```python
from build123d import *

# Parameters (mm, degrees)
SKETCH2_R          = 4
CUT_EXTRUDE1_DEPTH = 39.594040991
SKETCH3_R          = 1.5
CUT_EXTRUDE2_DEPTH = 39.594040991
CIRPATTERN1_COUNT  = 2
CIRPATTERN1_ANGLE  = 90
CUT_EXTRUDE3_DEPTH = 26
FILLET2_R          = 1
CIRPATTERN2_START  = 1.5
CIRPATTERN2_DEPTH  = 26


# Read off the part's stored shape, not the designer's step: CirPattern2
with BuildPart() as part:
    # Sketch1 → Revolve1 (revolve)
    with BuildSketch(Plane.XY, mode=Mode.PRIVATE) as revolve1_sk:
        Polygon((0, 0), (0, 11.5), (1.5, 11.5), (1.5, 9.5), (27.5, 9.5), (27.5, 11.5), (29, 11.5), (29, 6.5), (35, 6.5), (35, 0), align=None)
    revolve(revolve1_sk.sketch.rotate(Axis((-4.735156117, 0, 0), (1, 0, 0)), 90), axis=Axis((-4.735156117, 0, 0), (1, 0, 0)))

    # Sketch2 → Cut-Extrude1 (cut, through all)
    with BuildSketch(Plane.ZY):
        Circle(SKETCH2_R)
    extrude(amount=-CUT_EXTRUDE1_DEPTH, mode=Mode.SUBTRACT)

    # Sketch3 → Cut-Extrude2 (cut, through all)
    with BuildSketch(Plane(origin=(0, 0, 0), x_dir=(1, 0, 0), z_dir=(0, 1, 0))):
        with Locations(Location((32, 0, 0), (0, 0, 90))):
            Circle(SKETCH3_R)
    cut_extrude2 = extrude(amount=CUT_EXTRUDE2_DEPTH, mode=Mode.SUBTRACT)

    # CirPattern1: Cut-Extrude2 ×2 about axis
    cirpattern1_axis = Axis((-4.735156117, 0, 0), (-1, 0, 0))
    for i in range(1, CIRPATTERN1_COUNT):
        add(cut_extrude2.rotate(cirpattern1_axis, i * CIRPATTERN1_ANGLE / (CIRPATTERN1_COUNT - 1)), mode=Mode.SUBTRACT)

    # Sketch4 → Cut-Extrude3 (cut)
    with BuildSketch(Plane(origin=(1.5, 0, 0), x_dir=(0, 0, -1), z_dir=(1, 0, 0))):
        Polygon((2, 11.5), (-2, 11.5), (-1, 7.5), (1, 7.5), align=None)
    extrude(amount=CUT_EXTRUDE3_DEPTH, mode=Mode.SUBTRACT)

    # Fillet2
    fillet2_edges = [part.edges().sort_by_distance(p)[0] for p in [
        (14.5, 7.5, -1),
        (14.5, 9.385369037, -1.471342259),
        (14.5, 9.385369037, 1.471342259),
        (14.5, 7.5, 1),
    ]]
    fillet(fillet2_edges, radius=FILLET2_R)

    # CirPattern2 outline → CirPattern2 (cut)
    with BuildSketch(Plane.YZ.offset(CIRPATTERN2_START)):
        with BuildLine():
            ThreePointArc((9.173931529, 2.467585925), (8.227241336, 4.75), (6.723957861, 6.711064794))
            ThreePointArc((6.723957861, 6.711064794), (7.00459855, 5.999230542), (6.6998571, 5.297375964))
            Line((6.6998571, 5.297375964), (6.556490873, 5.158753439))
            ThreePointArc((6.556490873, 5.158753439), (6.261292098, 4.578713089), (6.385578732, 3.939853201))
            Line((6.385578732, 3.939853201), (6.604802325, 3.560146799))
            ThreePointArc((6.604802325, 3.560146799), (7.095927901, 3.133081473), (7.745856966, 3.098710936))
            Line((7.745856966, 3.098710936), (7.937590709, 3.153558469))
            ThreePointArc((7.937590709, 3.153558469), (8.697785327, 3.066545017), (9.173931529, 2.467585925))
        make_face()
        with BuildLine():
            ThreePointArc((6.723957861, 6.711064794), (4.757893172, 8.22267916), (2.467585925, 9.173931529))
            ThreePointArc((2.467585925, 9.173931529), (3.066545017, 8.697785327), (3.153558469, 7.937590709))
            Line((3.153558469, 7.937590709), (3.098710936, 7.745856966))
            ThreePointArc((3.098710936, 7.745856966), (3.133081473, 7.095927901), (3.560146799, 6.604802325))
            Line((3.560146799, 6.604802325), (3.939853201, 6.385578732))
            ThreePointArc((3.939853201, 6.385578732), (4.578713089, 6.261292098), (5.158753439, 6.556490873))
            Line((5.158753439, 6.556490873), (5.297272586, 6.699750184))
            ThreePointArc((5.297272586, 6.699750184), (6.008242375, 7.004605475), (6.723957861, 6.711064794))
        make_face()
        with BuildLine():
            ThreePointArc((2.467585925, 9.173931529), (0.009116775, 9.499995625), (-2.449973668, 9.178650719))
            ThreePointArc((-2.449973668, 9.178650719), (-1.693186777, 9.065775559), (-1.237733608, 8.450934433))
            Line((-1.237733608, 8.450934433), (-1.189366094, 8.257464375))
            ThreePointArc((-1.189366094, 8.257464375), (-0.834635803, 7.711794562), (-0.219223594, 7.5))
            Line((-0.219223594, 7.5), (0.219223594, 7.5))
            ThreePointArc((0.219223594, 7.5), (0.834635803, 7.711794562), (1.189366094, 8.257464375))
            Line((1.189366094, 8.257464375), (1.237697538, 8.450790151))
            ThreePointArc((1.237697538, 8.450790151), (1.700987791, 9.070287472), (2.467585925, 9.173931529))
        make_face()
        with BuildLine():
            ThreePointArc((-2.449973668, 9.178650719), (-4.742102454, 8.231795935), (-6.711064795, 6.723957862))
            ThreePointArc((-6.711064795, 6.723957862), (-5.999230542, 7.00459855), (-5.297375964, 6.6998571))
            Line((-5.297375964, 6.6998571), (-5.158753439, 6.556490873))
            ThreePointArc((-5.158753439, 6.556490873), (-4.578713089, 6.261292098), (-3.939853201, 6.385578732))
            Line((-3.939853201, 6.385578732), (-3.560146799, 6.604802325))
            ThreePointArc((-3.560146799, 6.604802325), (-3.133081473, 7.095927901), (-3.098710936, 7.745856966))
            Line((-3.098710936, 7.745856966), (-3.153517566, 7.937447722))
            ThreePointArc((-3.153517566, 7.937447722), (-3.062045097, 8.705593266), (-2.449973668, 9.178650719))
        make_face()
        with BuildLine():
            ThreePointArc((-6.711064795, 6.723957862), (-8.22267916, 4.757893172), (-9.173931529, 2.467585925))
            ThreePointArc((-9.173931529, 2.467585925), (-8.697785327, 3.066545017), (-7.937590709, 3.153558469))
            Line((-7.937590709, 3.153558469), (-7.745856966, 3.098710936))
            ThreePointArc((-7.745856966, 3.098710936), (-7.095927901, 3.133081473), (-6.604802325, 3.560146799))
            Line((-6.604802325, 3.560146799), (-6.385578732, 3.939853201))
            ThreePointArc((-6.385578732, 3.939853201), (-6.261292098, 4.578713089), (-6.556490873, 5.158753439))
            Line((-6.556490873, 5.158753439), (-6.699750184, 5.297272586))
            ThreePointArc((-6.699750184, 5.297272586), (-7.004605475, 6.008242375), (-6.711064795, 6.723957862))
        make_face()
        with BuildLine():
            ThreePointArc((-9.173931529, 2.467585925), (-9.499995625, 0.009116775), (-9.178650719, -2.449973668))
            ThreePointArc((-9.178650719, -2.449973668), (-9.065775559, -1.693186777), (-8.450934433, -1.237733608))
            Line((-8.450934433, -1.237733608), (-8.257464375, -1.189366094))
            ThreePointArc((-8.257464375, -1.189366094), (-7.711794562, -0.834635803), (-7.5, -0.219223594))
            Line((-7.5, -0.219223594), (-7.5, 0.219223594))
            ThreePointArc((-7.5, 0.219223594), (-7.711794562, 0.834635803), (-8.257464375, 1.189366094))
            Line((-8.257464375, 1.189366094), (-8.450790151, 1.237697538))
            ThreePointArc((-8.450790151, 1.237697538), (-9.070287472, 1.700987791), (-9.173931529, 2.467585925))
        make_face()
        with BuildLine():
            ThreePointArc((-9.178650719, -2.449973668), (-8.231795935, -4.742102454), (-6.723957862, -6.711064795))
            ThreePointArc((-6.723957862, -6.711064795), (-7.00459855, -5.999230542), (-6.6998571, -5.297375964))
            Line((-6.6998571, -5.297375964), (-6.556490873, -5.158753439))
            ThreePointArc((-6.556490873, -5.158753439), (-6.261292098, -4.578713089), (-6.385578732, -3.939853201))
            Line((-6.385578732, -3.939853201), (-6.604802325, -3.560146799))
            ThreePointArc((-6.604802325, -3.560146799), (-7.095927901, -3.133081473), (-7.745856966, -3.098710936))
            Line((-7.745856966, -3.098710936), (-7.937447722, -3.153517566))
            ThreePointArc((-7.937447722, -3.153517566), (-8.705593266, -3.062045097), (-9.178650719, -2.449973668))
        make_face()
        with BuildLine():
            ThreePointArc((-6.723957862, -6.711064795), (-4.757893172, -8.22267916), (-2.467585925, -9.173931529))
            ThreePointArc((-2.467585925, -9.173931529), (-3.066545017, -8.697785327), (-3.153558469, -7.937590709))
            Line((-3.153558469, -7.937590709), (-3.098710936, -7.745856966))
            ThreePointArc((-3.098710936, -7.745856966), (-3.133081473, -7.095927901), (-3.560146799, -6.604802325))
            Line((-3.560146799, -6.604802325), (-3.939853201, -6.385578732))
            ThreePointArc((-3.939853201, -6.385578732), (-4.578713089, -6.261292098), (-5.158753439, -6.556490873))
            Line((-5.158753439, -6.556490873), (-5.297272586, -6.699750184))
            ThreePointArc((-5.297272586, -6.699750184), (-6.008242375, -7.004605475), (-6.723957862, -6.711064795))
        make_face()
        with BuildLine():
            ThreePointArc((-2.467585925, -9.173931529), (-0.009116775, -9.499995625), (2.449973668, -9.178650719))
            ThreePointArc((2.449973668, -9.178650719), (1.693186777, -9.065775559), (1.237733608, -8.450934433))
            Line((1.237733608, -8.450934433), (1.189366094, -8.257464375))
            ThreePointArc((1.189366094, -8.257464375), (0.834635803, -7.711794562), (0.219223594, -7.5))
            Line((0.219223594, -7.5), (-0.219223594, -7.5))
            ThreePointArc((-0.219223594, -7.5), (-0.834635803, -7.711794562), (-1.189366094, -8.257464375))
            Line((-1.189366094, -8.257464375), (-1.237697538, -8.450790151))
            ThreePointArc((-1.237697538, -8.450790151), (-1.700987791, -9.070287472), (-2.467585925, -9.173931529))
        make_face()
        with BuildLine():
            ThreePointArc((2.449973668, -9.178650719), (4.742102454, -8.231795935), (6.711064794, -6.723957861))
            ThreePointArc((6.711064794, -6.723957861), (5.999230542, -7.00459855), (5.297375964, -6.6998571))
            Line((5.297375964, -6.6998571), (5.158753439, -6.556490873))
            ThreePointArc((5.158753439, -6.556490873), (4.578713089, -6.261292098), (3.939853201, -6.385578732))
            Line((3.939853201, -6.385578732), (3.560146799, -6.604802325))
            ThreePointArc((3.560146799, -6.604802325), (3.133081473, -7.095927901), (3.098710936, -7.745856966))
            Line((3.098710936, -7.745856966), (3.153517566, -7.937447722))
            ThreePointArc((3.153517566, -7.937447722), (3.062045097, -8.705593266), (2.449973668, -9.178650719))
        make_face()
        with BuildLine():
            Line((6.556490873, -5.158753439), (6.699750184, -5.297272586))
            ThreePointArc((6.699750184, -5.297272586), (7.004605475, -6.008242375), (6.711064795, -6.723957862))
            ThreePointArc((6.711064795, -6.723957862), (8.22267916, -4.757893172), (9.173931529, -2.467585925))
            ThreePointArc((9.173931529, -2.467585925), (8.697785327, -3.066545017), (7.937590709, -3.153558469))
            Line((7.937590709, -3.153558469), (7.745856966, -3.098710936))
            ThreePointArc((7.745856966, -3.098710936), (7.095927901, -3.133081473), (6.604802325, -3.560146799))
            Line((6.604802325, -3.560146799), (6.385578732, -3.939853201))
            ThreePointArc((6.385578732, -3.939853201), (6.261292098, -4.578713089), (6.556490873, -5.158753439))
        make_face()
    extrude(amount=CIRPATTERN2_DEPTH, mode=Mode.SUBTRACT)


solid = part.part
```
Part model, mm, in its own coordinate system. A direction names the side the tool comes from. Round coordinates to 2 decimals unless told otherwise and drop trailing zeros. Loops run counter-clockwise (first coordinate to the right, second up) from the corner with the lowest first, then second, coordinate; pieces in that order, holes last. Notation, with made-up numbers: (-22.5, -13.75) -> (-18.5, -13.75) arc R23 ccw to (-18.5, 10.25) -> close; hole circle Ø6 at (-27, 28.25). An arc over 180 degrees is marked (long way). Use one line per item in the form item = value. Start each with the question number.
Item 1: Band-saw the part on C-C (z = 4.5). List the corners of the cut face in (x, y), plus the area to 3 significant figures.
Item 2: Band-saw the part on A-A (y = 10.25). List the corners of the cut face in (x, z).
Item 3: Band-saw the part on B-B (x = 32). List the corners of the cut face in (y, z), plus the area to 3 significant figures.
Item 4: Tool access for faces 4 (the cylindrical face through (14.318, 7.087, 3.137)), 5 (the cylindrical face through (14.318, -8.696, -3.067)), 6 (the cylindrical face through (14.32, -7.71, 0.83)): list every direction of +Z, -Z, +X, -X, +Y, -Y with a clear straight run to the whole face (end or side of a thin tool).
Item 5: Drop flat-ended pins along their axis: pin 1 Ø5 at (x, y) = (32, 0) entering from -Z; pin 2 Ø1.5 at (x, y) = (22.5, 6.5) entering from +Z; pin 3 Ø1.5 at (x, y) = (29.5, 1.5) entering from +Z; pin 4 Ø11.5 at (y, z) = (-2, 2) entering from -X. Give the stop position or say it passes through.
Item 6: Drill centre lines: line 1 along Z through (x, y) = (21.5, 0); line 2 along X through (y, z) = (4.4, 0); line 3 along X through (y, z) = (8.5, -6). Where is each one in solid material? Low to high.
Item 7: Two-plate mould, pull along X, no slides. Class faces 1 (the flat face through (0, 0, -5)), 2 (the cylindrical face through (14.318, -6.01, 7.005)), 3 (the cylindrical face through (0.8, -11.4, -1.5)): released by +X, released by -X, zero draft, split by the parting line, or undercut.
Data:
q1.outline = (0, -10.58) -> (1.5, -10.58) -> (1.5, -6.25) -> (27.5, -6.25) -> (27.5, -10.58) -> (29, -10.58) -> (29, -4.69) -> (35, -4.69) -> (35, 4.69) -> (29, 4.69) -> (29, 10.58) -> (27.5, 10.58) -> (27.5, 6.25) -> (1.5, 6.25) -> (1.5, 10.58) -> (0, 10.58) -> close
q1.area = 445 mm^2
q2.outline = (0, -5.21) -> (1.5, -5.21) -> (1.5, 5.21) -> (0, 5.21) -> close; (27.5, -5.21) -> (29, -5.21) -> (29, 5.21) -> (27.5, 5.21) -> close
q3.outline = (-1.5, -6.32) -> (-1.5, -3.71) arc R4 cw (long way) to (3.71, 1.5) -> (6.32, 1.5) arc R6.5 ccw (long way) to start; (1.5, -6.32) arc R6.5 ccw to (6.32, -1.5) -> (3.71, -1.5) arc R4 cw to (1.5, -3.71) -> close
q3.area = 67.2 mm^2
q4.face_4 = none
q4.face_5 = -Z
q4.face_6 = -Y
q5.pin_1 = -6.5
q5.pin_2 = 7
q5.pin_3 = 11.46
q5.pin_4 = 0
q6.line_1 = -7.5 to -4, 4 to 7.5
q6.line_2 = 0 to 30.5, 33.5 to 35
q6.line_3 = 0 to 1.5, 27.5 to 29
q7.face_1 = released by -X
q7.face_2 = undercut
q7.face_3 = zero draft
